For this review, take the finished solid that the model builds, in its own axes (mm). A direction names the side the tool comes from. Give positions to 0.01 mm unless a question says otherwise; leave off trailing zeros. Loops run counter-clockwise (first coordinate to the right, second up) from the corner with the lowest first, then second, coordinate; pieces in that order, holes last. Notation, with made-up numbers: (-6, -37) - (44, -37) arc R31 cw to (44, -13) - close; hole circle Ø2 at (11, 72.25). An arc over 180 degrees is marked (long way). Put each result on its own line as item: value.
from build123d import *

# Parameters (mm, degrees)
SKETCH1_R           = 180
BOSS_EXTRUDE1_DEPTH = 200
CUT_EXTRUDE1_DEPTH  = 80
SKETCH6_R           = 35.432069659
CUT_EXTRUDE4_DEPTH  = 201
SKETCH7_R           = 149.510464434
SKETCH7_R_2         = 139.963931463
SKETCH7_R_3         = 102.629519035
SKETCH7_R_4         = 93.728776548
CUT_EXTRUDE6_DEPTH  = 30
CUT_EXTRUDE7_START  = 190
SKETCH8_R           = 58.778682825
CUT_EXTRUDE7_DEPTH  = 30
CUT_EXTRUDE8_START  = -150
SKETCH9_R           = 58.778682825
CUT_EXTRUDE8_DEPTH  = 236


with BuildPart() as part:
    # Sketch1 → Boss-Extrude1 (new body)
    with BuildSketch(Plane.XY):
        Circle(SKETCH1_R)
    extrude(amount=BOSS_EXTRUDE1_DEPTH)

    # Sketch2 → Cut-Extrude1 (cut)
    with BuildSketch(Plane(origin=(0, 0, 0), x_dir=(-1, 0, 0), z_dir=(0, 0, -1))):
        Polygon((50, -50), (50, -249.832537204), (-50, -249.832537204), (-50, -50), (-236.119265231, -50), (-236.119265231, 53.613723388), (-50, 53.613723388), (-50, 228.035589712), (50, 228.035589712), (50, 53.613723388), (294.314355645, 53.613723388), (294.314355645, -50), align=None)
    extrude(amount=-CUT_EXTRUDE1_DEPTH, mode=Mode.SUBTRACT)

    # Sketch6 → Cut-Extrude4 (cut, through all)
    with BuildSketch(Plane(origin=(0, 0, 0), x_dir=(-1, 0, 0), z_dir=(0, 0, -1))):
        Circle(SKETCH6_R)
    extrude(amount=-CUT_EXTRUDE4_DEPTH, mode=Mode.SUBTRACT)

    # Sketch7 → Cut-Extrude6 (cut)
    with BuildSketch(Plane(origin=(0, 0, 0), x_dir=(-1, 0, 0), z_dir=(0, 0, -1))):
        Circle(SKETCH7_R)
        Circle(SKETCH7_R_2, mode=Mode.SUBTRACT)
        Circle(SKETCH7_R_3)
        Circle(SKETCH7_R_4, mode=Mode.SUBTRACT)
    extrude(amount=-CUT_EXTRUDE6_DEPTH, mode=Mode.SUBTRACT)

    # Sketch8 → Cut-Extrude7 (cut)
    with BuildSketch(Plane(origin=(0, 0, 0), x_dir=(0, 0, -1), z_dir=(1, 0, 0)).offset(CUT_EXTRUDE7_START)):
        with Locations((-120.694647065, 0)):
            Circle(SKETCH8_R)
    extrude(amount=-CUT_EXTRUDE7_DEPTH, mode=Mode.SUBTRACT)

    # Sketch9 → Cut-Extrude8 (cut)
    with BuildSketch(Plane(origin=(0, 0, 0), x_dir=(0, 0, -1), z_dir=(1, 0, 0)).offset(CUT_EXTRUDE8_START)):
        with Locations((-120.694647065, 0)):
            Circle(SKETCH9_R)
    extrude(amount=-CUT_EXTRUDE8_DEPTH, mode=Mode.SUBTRACT)


solid = part.part
1) Wall thickness on line 1 (X direction, y = -61.5, z = 29); line 2 (Y direction, x = -106, z = 28.5); line 3 (X direction, y = -42.5, z = 126.5): over which ranges is each line inside the solid? List them lowest first.
Geometry check:
line 1: x = -169.17 to -136.28, -125.73 to -82.16, -70.73 to -50, 50 to 70.73, 82.16 to 125.73, 136.28 to 169.17
line 2: y = -145.48 to -105.44, -91.4 to -50, 53.61 to 91.4, 105.44 to 145.48
line 3: x = -150 to 160
2) Draft analysis for pull direction Y (two halves, no side actions). For faces 1 (the face through (61, -61, 0)), 2 (the face through (-99, -102, 30)), state which applies: pulls with the +Y half, pulls with the -Y half, needs draft (parallel to the pull), parting line crosses it, or undercut.
Geometry check:
face 1: needs draft
face 2: undercut
3) Insertion check: pin 1 Ø6 at (y, z) = (7.5, 87.5) entering from -X; pin 2 Ø18 at (x, y) = (-71, 74) entering from -Z; pin 3 Ø6 at (y, z) = (43, 155) entering from +X; pin 4 Ø24 at (y, z) = (105.5, 59.5) entering from -X. Each pin has a flat end and moves straight along its axis. Give the tip position at first contact, or say it passes through.
Geometry check:
pin 1: stops at x = -150
pin 2: stops at z = 0
pin 3: stops at x = 160
pin 4: stops at x = -153.81
4) Take a section at D-D on z = 152.5. State the section outline as (x, y) points.
Geometry check:
outline: (-173.08, -49.43) arc R180 ccw to (173.08, -49.43) - (160, -49.43) - (160, 49.43) - (173.08, 49.43) arc R180 ccw to (-173.08, 49.43) - (-150, 49.43) - (-150, -49.43) - close; hole circle Ø70.86 at (0, 0)
5) Take a section at A-A on y = 0. State the section outline as (x, z) points, and give its area (3 significant figures).
Geometry check:
outline: (-180, 179.47) - (-150, 179.47) - (-150, 80) - (-35.43, 80) - (-35.43, 200) - (-180, 200) - close; (35.43, 80) - (160, 80) - (160, 179.47) - (180, 179.47) - (180, 200) - (35.43, 200) - close
area: 29,700 mm²
6) Take a section at B-B on x = 0. State the section outline as (y, z) points, and give its area (3 significant figures).
Geometry check:
outline: (-180, 80) - (-35.43, 80) - (-35.43, 200) - (-180, 200) - close; (35.43, 80) - (180, 80) - (180, 200) - (35.43, 200) - close
area: 34,700 mm²
7) Take a section at C-C on z = 48. State the section outline as (x, y) points.
Geometry check:
outline: (-172.92, -50) arc R180 ccw to (-50, -172.92) - (-50, -50) - close; (-171.83, 53.61) - (-50, 53.61) - (-50, 172.92) arc R180 ccw to start; (50, -172.92) arc R180 ccw to (172.92, -50) - (50, -50) - close; (50, 53.61) - (171.83, 53.61) arc R180 ccw to (50, 172.92) - close
8) For faces 3 (the face through (72.85, -72.29, 14.79)), 4 (the face through (-110, 53.614, 39)), 5 (the face through (167.92, 1.92, 179.44)), list the 3-axis set-ups (+Z, -Z, +X, -X, +Y, -Y) from which the entire face can be reached by the end or side of a thin tool; tool diameter is ignored.
Geometry check:
face 3: -Z
face 4: -Z, +X, -X
face 5: +X
